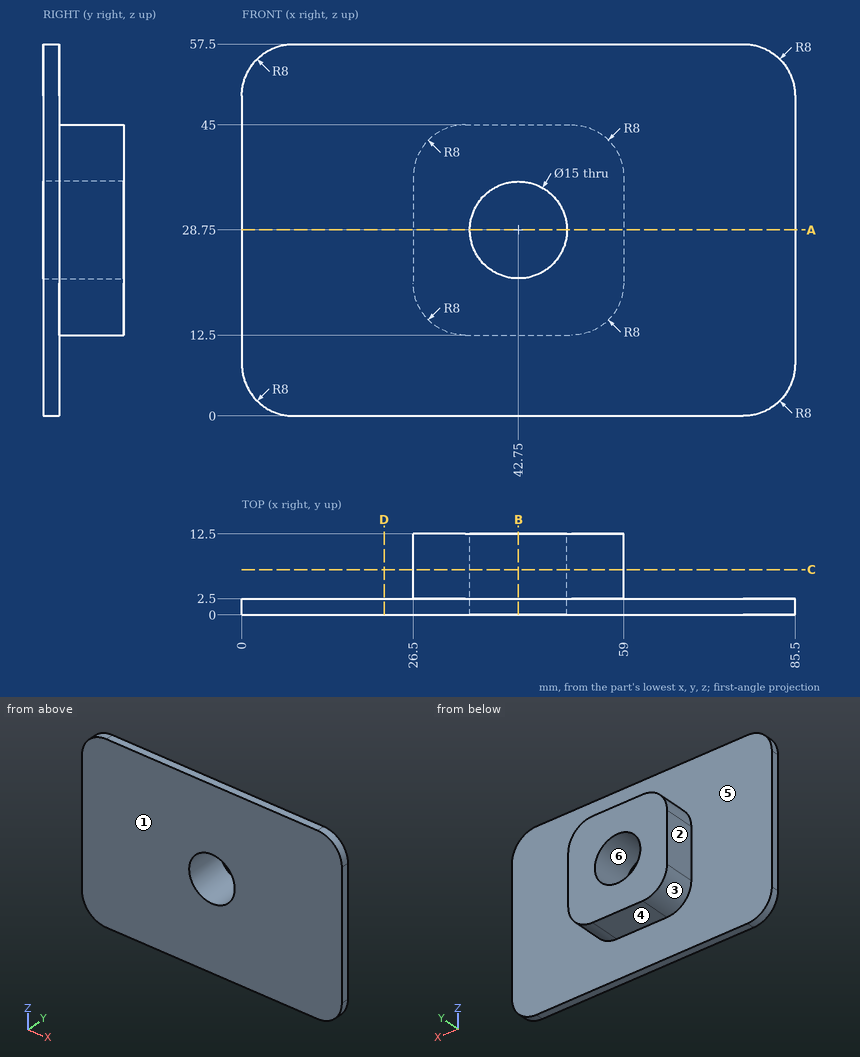
The drawing under review shows one solid part. Ordinate dimensions are in mm from its lowest x, y, z. A direction names the side the tool comes from. Round coordinates to 2 decimals unless told otherwise and drop trailing zeros. Write each loop counter-clockwise with the first axis right and the second up, starting at its lowest first coordinate (ties: lowest second). Pieces come first, ordered by that corner, then holes. Notation, with made-up numbers: (-30, 5.25) -> (13, 5.25) arc R16 cw to (13, 9.25) -> close; hole circle Ø7 at (-21.75, 40). An arc over 180 degrees is marked (long way). One line per question, with ' | ' between items. Start each with the question number.
(1) Add section C-C, the plane y = 7. Write out the cut boundary in (x, z).
(2) Add section D-D, the plane x = 22. Write out the cut boundary in (y, z), plus the area to 3 significant figures.
(3) For line 1 along X through (y, z) = (9.5, 28.75); line 2 along Z through (x, y) = (78, 1); line 3 along Y through (x, z) = (64.5, 18), list the stretches that pass through material, from the lowest coordinate up. Write a range as from..to.
(4) Mouldability with a two-part tool opening along Z and no side actions: class the marked faces 4, 5 and 6 as released by +Z, released by -Z, zero draft, split by the parting line, or undercut.
(5) Add section A-A, the plane z = 28.75. Write out the cut boundary in (x, y), plus the area to 3 significant figures.
(6) Add section B-B, the plane x = 42.75. Write out the cut boundary in (y, z).
(7) Insertion check: P1, Ø1.5, axis at y = 5.5, z = 22, coming from the +X side; P2, Ø10, axis at x = 18, z = 39, coming from the +Y side; P3, Ø3, axis at x = 39, y = 6.5, coming from the +Z side. Each pin has a flat end and moves straight along its axis. Give the tip position at first contact, or say it passes through.
(8) Tool access review of the marked faces 1, 2 and 3: name each direction out of +Z, -Z, +X, -X, +Y, -Y from which nothing blocks a thin tool from reaching the whole face with its end or side.
Answer list:
1) outline: (26.5, 20.5) arc R8 ccw to (34.5, 12.5) -> (51, 12.5) arc R8 ccw to (59, 20.5) -> (59, 37) arc R8 ccw to (51, 45) -> (34.5, 45) arc R8 ccw to (26.5, 37) -> close; hole circle Ø15 at (42.75, 28.75)
2) outline: (0, 0) -> (2.5, 0) -> (2.5, 57.5) -> (0, 57.5) -> close | area: 144 mm²
3) line 1: 26.5..35.25, 50.25..59 | line 2: 0.02..57.48 | line 3: 0..2.5
4) face 4: released by -Z | face 5: zero draft | face 6: undercut
5) outline: (0, 0) -> (35.25, 0) -> (35.25, 12.5) -> (26.5, 12.5) -> (26.5, 2.5) -> (0, 2.5) -> close; (50.25, 0) -> (85.5, 0) -> (85.5, 2.5) -> (59, 2.5) -> (59, 12.5) -> (50.25, 12.5) -> close | area: 351 mm²
6) outline: (0, 0) -> (2.5, 0) -> (2.5, 12.5) -> (12.5, 12.5) -> (12.5, 21.25) -> (0, 21.25) -> close; (0, 36.25) -> (12.5, 36.25) -> (12.5, 45) -> (2.5, 45) -> (2.5, 57.5) -> (0, 57.5) -> close
7) P1: x = 59 | P2: y = 2.5 | P3: z = 45
8) face 1: +Z, -Z, +X, -X, -Y | face 2: +Z, -Z, -X, +Y | face 3: -Z, -X, +Y
